Read the model definition and answer for the solid it produces. Units are mm, in the model's axes. A direction names the side the tool comes from. Coordinates: 2 decimals unless noted, no trailing zeros. Write each loop counter-clockwise with the first axis right and the second up, starting at its lowest first coordinate (ties: lowest second). Pieces come first, ordered by that corner, then holes.
1) Each of these flat-tipped pins is pushed along its axis until it touches: pin 1 Ø2 at (x, z) = (5.5, -14.5) entering from +Y; pin 2 Ø4 at (x, z) = (63.5, 26.38) entering from -Y. Where does it stop, or does it pass through?
2) Find the intervals of material crossed by line 1 (X direction, y = 5, z = -16.1); line 2 (X direction, y = 7.5, z = 12.9); line 3 (Z direction, x = -62.5, y = 6.25), in increasing order.
3) Determine the mould class of faces 4 (the face through (69.85, 5, 12)), 5 (the face through (-69.85, 5, 12)), 6 (the face through (7, 6.726, 14)) for opening direction X: +X half, -X half, draft (parallel to the pull), parting line (faces both ways), or undercut.
4) Which of the six approach directions +Z, -Z, +X, -X, +Y, -Y give full straight-line access (tool end or side, diameter ignored) to faces 1 (the face through (7, 6.726, -15)), 2 (the face through (-64, 2.799, 25)), 3 (the face through (64.55, 6.11, 25.7))?
5) The part is cut by section A-A (z = 0). Determine the outline of the cut face in (x, y) (3 decimals), then the cut area to 3 significant figures.
6) The part is cut by section B-B (z = 12.9). Determine the outline of the cut face in (x, y) (3 decimals).
from build123d import *

# Parameters (mm, degrees)
SKETCH1_W           = 139.7
SKETCH1_H           = 50.8
BOSS_EXTRUDE1_DEPTH = 9.525
SKETCH13_W          = 139.7
SKETCH13_H          = 9.525
BOSS_EXTRUDE2_DEPTH = 25.4
SKETCH45_R          = 2.77495
CUT_EXTRUDE3_DEPTH  = 2.79908
SKETCH47_R          = 1.25
CUT_EXTRUDE4_DEPTH  = 87.892969365
SKETCH2_R           = 1.65
CUT_EXTRUDE5_DEPTH  = 87.892969365
SKETCH50_R          = 3.52552
CUT_EXTRUDE6_DEPTH  = 2.79908
SKETCH51_R          = 1.25
CUT_EXTRUDE10_DEPTH = 87.892969365
SKETCH35_R          = 1.25
CUT_EXTRUDE11_DEPTH = 87.892969365


with BuildPart() as part:
    # Sketch1 → Boss-Extrude1 (new body)
    with BuildSketch(Plane(origin=(0, 0, 0), x_dir=(1, 0, 0), z_dir=(0, 1, 0))):
        Rectangle(SKETCH1_W, SKETCH1_H)
    extrude(amount=BOSS_EXTRUDE1_DEPTH)

    # Sketch13 → Boss-Extrude2 (add)
    with BuildSketch(Plane.XY.offset(25.4)):
        with Locations((0, 4.7625)):
            Rectangle(SKETCH13_W, SKETCH13_H)
    extrude(amount=BOSS_EXTRUDE2_DEPTH)

    # Sketch45 → Cut-Extrude3 (cut)
    with BuildSketch(Plane.XZ):
        with Locations(Location((63.5, 26.37536, 0), (0, 0, 270))):
            Circle(SKETCH45_R)
        with Locations(Location((-63.5, 26.37536, 0), (0, 0, 270))):
            Circle(SKETCH45_R)
    extrude(amount=-CUT_EXTRUDE3_DEPTH, mode=Mode.SUBTRACT)

    # Sketch47 → Cut-Extrude4 (cut, through all)
    with BuildSketch(Plane.XZ):
        with Locations(Location((63.5, 26.37536, 0), (0, 0, 270))):
            Circle(SKETCH47_R)
        with Locations(Location((-63.5, 26.37536, 0), (0, 0, 270))):
            Circle(SKETCH47_R)
    extrude(amount=-CUT_EXTRUDE4_DEPTH, mode=Mode.SUBTRACT)

    # Sketch2 → Cut-Extrude5 (cut, through all)
    with BuildSketch(Plane(origin=(0, 9.525, 0), x_dir=(1, 0, 0), z_dir=(0, 1, 0))):
        with Locations(Location((-9.906, 16.1, 0), (0, 0, 270))):
            Circle(SKETCH2_R)
        with Locations(Location((5.094, 16.1, 0), (0, 0, 270))):
            Circle(SKETCH2_R)
        with Locations(Location((-9.906, -12.9, 0), (0, 0, 270))):
            Circle(SKETCH2_R)
        with Locations(Location((5.094, -12.9, 0), (0, 0, 270))):
            Circle(SKETCH2_R)
        with Locations(Location((-59.5, 0, 0), (0, 0, 270))):
            Circle(SKETCH2_R)
        with Locations(Location((59.5, 0, 0), (0, 0, 270))):
            Circle(SKETCH2_R)
    extrude(amount=-CUT_EXTRUDE5_DEPTH, mode=Mode.SUBTRACT)

    # Sketch50 → Cut-Extrude6 (cut)
    with BuildSketch(Plane(origin=(0, 9.525, 0), x_dir=(1, 0, 0), z_dir=(0, 1, 0))):
        with Locations(Location((-9.906, 16.1, 0), (0, 0, 270))):
            Circle(SKETCH50_R)
        with Locations(Location((5.094, 16.1, 0), (0, 0, 270))):
            Circle(SKETCH50_R)
        with Locations(Location((5.094, -12.9, 0), (0, 0, 270))):
            Circle(SKETCH50_R)
        with Locations(Location((-9.906, -12.9, 0), (0, 0, 270))):
            Circle(SKETCH50_R)
    extrude(amount=-CUT_EXTRUDE6_DEPTH, mode=Mode.SUBTRACT)

    # Sketch51 → Cut-Extrude10 (cut, through all)
    with BuildSketch(Plane(origin=(0, 9.525, 0), x_dir=(1, 0, 0), z_dir=(0, 1, 0))):
        with Locations(Location((-63.5, 22.06371, 0), (0, 0, 270))):
            Circle(SKETCH51_R)
        with Locations(Location((63.5, 22.06371, 0), (0, 0, 270))):
            Circle(SKETCH51_R)
    extrude(amount=-CUT_EXTRUDE10_DEPTH, mode=Mode.SUBTRACT)

    # Sketch35 → Cut-Extrude11 (cut, through all)
    with BuildSketch(Plane(origin=(0, 0, 0), x_dir=(1, 0, 0), z_dir=(0, 1, 0))):
        with Locations(Location((9.525, -34.9, 0), (0, 0, 90))):
            Circle(SKETCH35_R)
        with Locations(Location((-9.525, -34.9, 0), (0, 0, 90))):
            Circle(SKETCH35_R)
        with Locations(Location((-9.525, -42.85, 0), (0, 0, 90))):
            Circle(SKETCH35_R)
        with Locations(Location((9.525, -42.85, 0), (0, 0, 90))):
            Circle(SKETCH35_R)
    extrude(amount=CUT_EXTRUDE11_DEPTH, mode=Mode.SUBTRACT)


solid = part.part
Reported:
1. pin 1: stops at y = 6.73
1. pin 2: stops at y = 2.8
2. line 1: x = -69.85 to -11.56, -8.26 to 3.44, 6.74 to 69.85
2. line 2: x = -69.85 to -13.43, -6.38 to 1.57, 8.62 to 69.85
2. line 3: z = -25.4 to -22.81, -21.31 to 25.63, 27.13 to 50.8
3. face 4: +X half
3. face 5: -X half
3. face 6: undercut
4. face 1: +Y
4. face 2: -Y
4. face 3: +Y, -Y
5. outline: (-69.85, 0) - (-61.15, 0) - (-61.15, 9.525) - (-69.85, 9.525) - close; (-57.85, 0) - (57.85, 0) - (57.85, 9.525) - (-57.85, 9.525) - close; (61.15, 0) - (69.85, 0) - (69.85, 9.525) - (61.15, 9.525) - close
5. area: 1,270 mm2
6. outline: (-69.85, 0) - (-11.556, 0) - (-11.556, 6.726) - (-13.432, 6.726) - (-13.432, 9.525) - (-69.85, 9.525) - close; (-8.256, 0) - (3.444, 0) - (3.444, 6.726) - (1.568, 6.726) - (1.568, 9.525) - (-6.38, 9.525) - (-6.38, 6.726) - (-8.256, 6.726) - close; (6.744, 0) - (69.85, 0) - (69.85, 9.525) - (8.62, 9.525) - (8.62, 6.726) - (6.744, 6.726) - close
